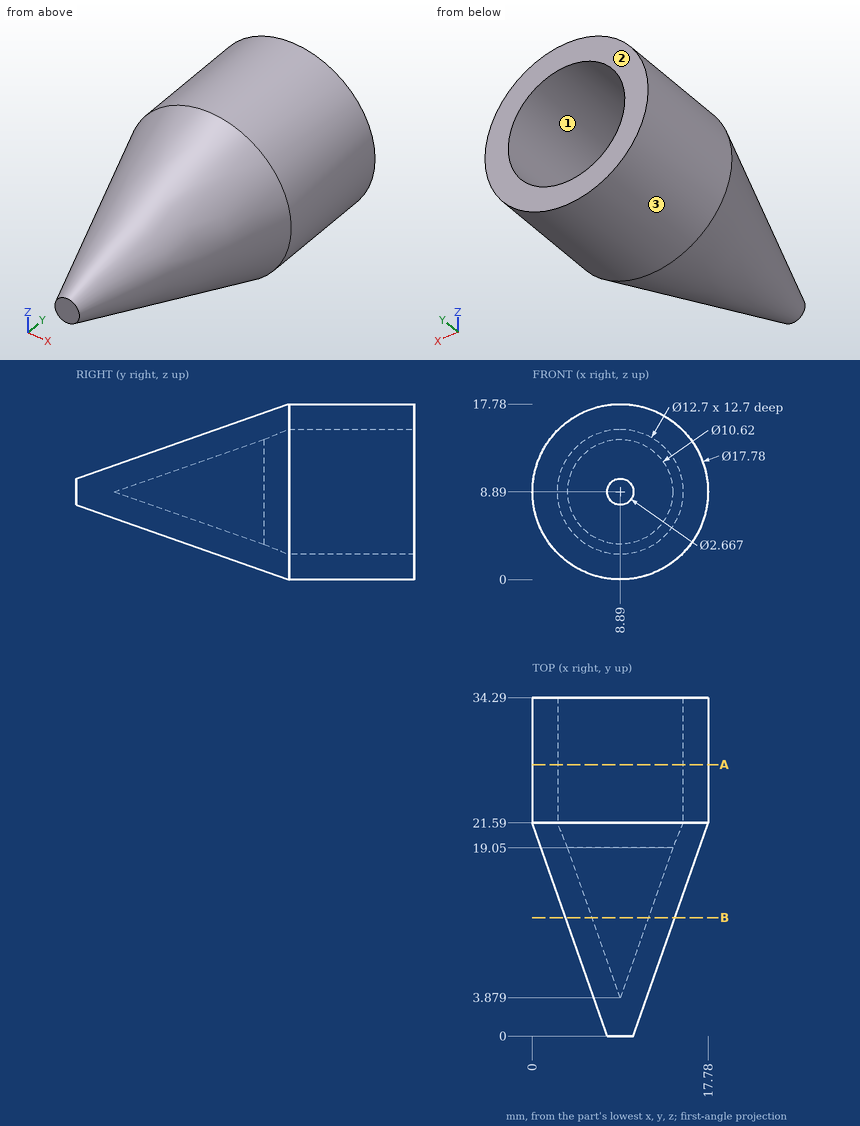
Geometry check sheet. Reference: drawing and pictorial views, mm from the part's lowest x, y, z. Round coordinates to 2 decimals unless told otherwise and drop trailing zeros. Write each loop counter-clockwise with the first axis right and the second up, starting at its lowest first coordinate (ties: lowest second). Pieces come first, ordered by that corner, then holes.
1. Draft check along Z on the marked faces 1, 2 and 3. Enter one of: +Z half, -Z half, draft (parallel to the pull), parting line (faces both ways), or undercut.
2. Section check A-A on y = 27.5. Enter the section's corners in (x, z), plus the area to 3 significant figures.
3. Scan lines: L1, parallel to X at y = 25.75, z = 8.89; L2, parallel to Z at x = 11, y = 18. Record each from-to range of solid material in increasing order.
4. Gauge pin test, flat ends, axial feed: P1, Ø1.5, axis at x = 14.5, y = 9.5, coming from the -Z side; P2, Ø6, axis at x = 14, y = 30.5, coming from the +Z side; P3, Ø2, axis at x = 3, y = 27, coming from the +Z side; P4, Ø2, axis at y = 17.5, z = 15, coming from the -X side. Record the tip position at first contact, or that the pin passes through.
5. Section check B-B on y = 12. Enter the section's corners in (x, z) (1 decimal).
Answer:
1. face 1: undercut
1. face 2: draft
1. face 3: parting line
2. outline: circle Ø17.78 at (8.89, 8.89); hole circle Ø12.7 at (8.89, 8.89)
2. area: 122 mm2
3. L1: x = 0 to 2.54, 15.24 to 17.78
3. L2: z = 1.55 to 4.42, 13.36 to 16.23
4. P1: passes through
4. P2: stops at z = 17.53
4. P3: stops at z = 16.31
4. P4: stops at x = 3.34
5. outline: circle Ø11.1 at (8.9, 8.9); hole circle Ø5.7 at (8.9, 8.9)
